Part print with two shaded views. Sizes in mm from the minimum x, y, z corner. A direction names the side the tool comes from. Round coordinates to 2 decimals unless told otherwise and drop trailing zeros. Write each loop counter-clockwise with the first axis right and the second up, starting at its lowest first coordinate (ties: lowest second). Pieces come first, ordered by that corner, then holes. Notation, with made-up numbers: (-4, 46) -> (28, 46) arc R22 cw to (28, 85) -> close; hole circle Ø9 at (15, 25.5). An arc over 180 degrees is marked (long way). Return JSON: item names as keys, results as strings.
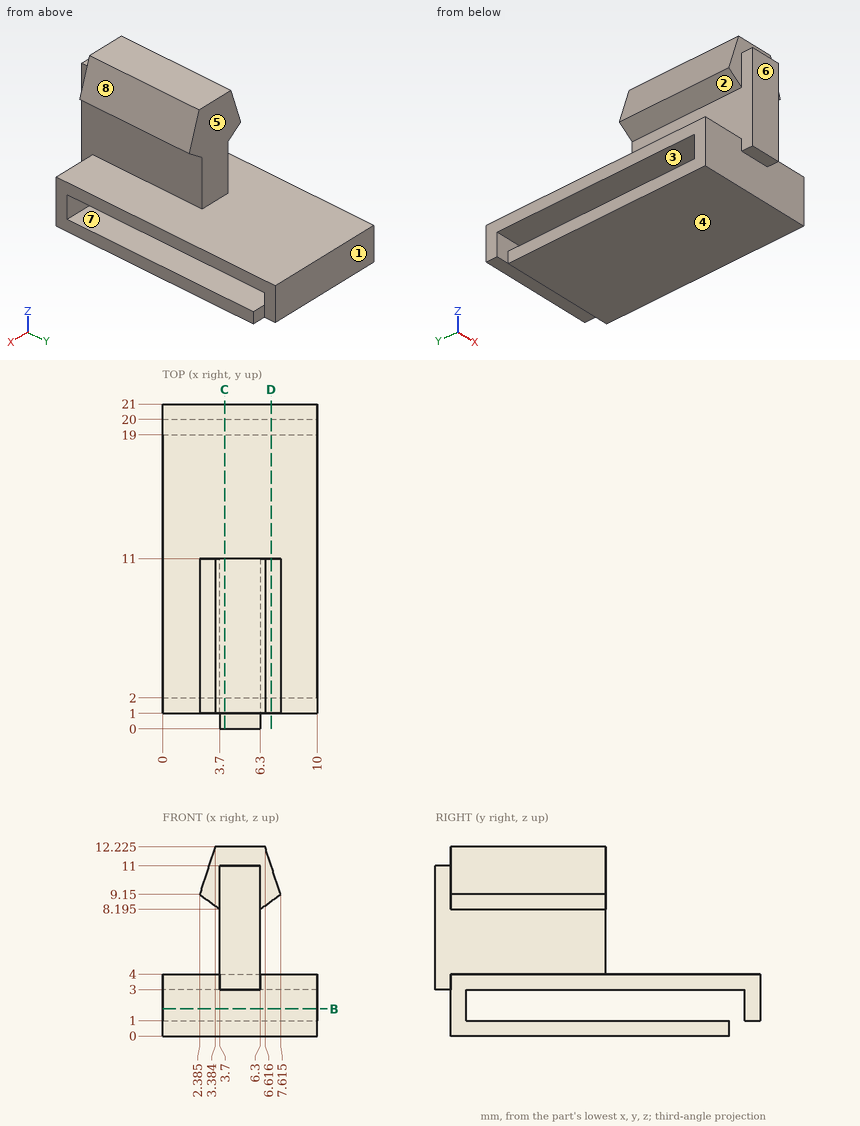
Q1. Two-plate mould, pull along Y, no slides. Class the marked faces 6, 7 and 8: +Y half, -Y half, draft (parallel to the pull), parting line (faces both ways), or undercut.
Verdict:
{"face 6": "-Y half", "face 7": "undercut", "face 8": "draft"}
Q2. Saw through at C-C on x = 4. List the corners of the cut face in (y, z) (1 decimal).
Verdict:
{"outline": "(0, 3) -> (1, 3) -> (1, 0) -> (19, 0) -> (19, 1) -> (2, 1) -> (2, 3) -> (20, 3) -> (20, 1) -> (21, 1) -> (21, 4) -> (11, 4) -> (11, 12.2) -> (1, 12.2) -> (1, 11) -> (0, 11) -> close"}
Q3. Saw through at D-D on x = 7. List the corners of the cut face in (y, z) (1 decimal).
Verdict:
{"outline": "(1, 0) -> (19, 0) -> (19, 1) -> (2, 1) -> (2, 3) -> (20, 3) -> (20, 1) -> (21, 1) -> (21, 4) -> (1, 4) -> close; (1, 8.7) -> (11, 8.7) -> (11, 11) -> (1, 11) -> close"}
Q4. 3-axis set-ups, long thin cutter, end or side, ignore diameter. For the marked faces 1, 2, 3, 4 and 5: which of +Z, -Z, +X, -X, +Y, -Y reach the whole face in a straight line?
Verdict:
{"face 1": "+Z, -Z, +X, -X, +Y", "face 2": "-X, +Y, -Y", "face 3": "+X, -X", "face 4": "-Z, +X, -X, +Y, -Y", "face 5": "+Z, +X, -X, +Y"}
Q5. Wall check: L1, parallel to Z at x = 1, y = 5; L2, parallel to Y at x = 4.5, z = 2.25; L3, parallel to Y at x = 6, z = 7.5. Give the ranges that are in metal, low to high.
Verdict:
{"L1": "z = 0 to 1, 3 to 4", "L2": "y = 1 to 2, 20 to 21", "L3": "y = 0 to 11"}
Q6. Pin check, flat tips, straight feed: pin 1 Ø6 at (y, z) = (8, 9) entering from +X (1 decimal); pin 2 Ø5 at (y, z) = (17.5, 2) entering from -X; pin 3 Ø0.8 at (x, y) = (5, 0.5) entering from +Z; pin 4 Ø3 at (x, z) = (3.5, 1) entering from -Y. Stop position of each tip, or through.
Verdict:
{"pin 1": "stops at x = 7.6", "pin 2": "stops at x = 0", "pin 3": "stops at z = 11", "pin 4": "stops at y = 1"}
Q7. Saw through at B-B on z = 1.75. List the corners of the cut face in (x, y).
Verdict:
{"outline": "(0, 1) -> (10, 1) -> (10, 2) -> (0, 2) -> close; (0, 20) -> (10, 20) -> (10, 21) -> (0, 21) -> close"}
